from build123d import *

# Parameters (mm, degrees)
SKETCH1_W            = 105
SKETCH1_H            = 85
BOSS_EXTRUDE1_DEPTH  = 3
SKETCH2_W            = 2.8
SKETCH2_H            = 2.8
BOSS_EXTRUDE2_DEPTH  = 15
SKETCH2_7_W          = 7
SKETCH2_7_H          = 7
SKETCH2_7_W_2        = 2.8
SKETCH2_7_H_2        = 2.8
BOSS_EXTRUDE3_DEPTH  = 10
SKETCH4_W            = 2.8
SKETCH4_H            = 2.8
BOSS_EXTRUDE7_DEPTH  = 15
SKETCH8_W            = 7
SKETCH8_H            = 7
SKETCH8_W_2          = 2.8
SKETCH8_H_2          = 2.8
BOSS_EXTRUDE8_DEPTH  = 10
SKETCH9_W            = 2.8
SKETCH9_H            = 2.8
BOSS_EXTRUDE9_DEPTH  = 15
SKETCH10_W           = 7
SKETCH10_H           = 7
SKETCH10_W_2         = 2.8
SKETCH10_H_2         = 2.8
BOSS_EXTRUDE10_DEPTH = 10


with BuildPart() as part:
    # Sketch1 → Boss-Extrude1 (new body)
    with BuildSketch(Plane(origin=(0, 0, 0), x_dir=(1, 0, 0), z_dir=(0, 1, 0))):
        with Locations((-10.290249703, -17.251010702)):
            Rectangle(SKETCH1_W, SKETCH1_H)
    extrude(amount=BOSS_EXTRUDE1_DEPTH)

    # Sketch2 → Boss-Extrude2 (add)
    with BuildSketch(Plane(origin=(0, 3, 0), x_dir=(1, 0, 0), z_dir=(0, 1, 0))):
        with Locations((-24.290249703, -56.430856566)):
            Rectangle(SKETCH2_W, SKETCH2_H)
    extrude(amount=BOSS_EXTRUDE2_DEPTH)

    # Sketch2<7> → Boss-Extrude3 (add)
    with BuildSketch(Plane(origin=(0, 3, 0), x_dir=(1, 0, 0), z_dir=(0, 1, 0))):
        with Locations((-24.290249703, -56.251010702)):
            Rectangle(SKETCH2_7_W, SKETCH2_7_H)
        with Locations((-24.290249703, -56.430856566)):
            Rectangle(SKETCH2_7_W_2, SKETCH2_7_H_2, mode=Mode.SUBTRACT)
    extrude(amount=BOSS_EXTRUDE3_DEPTH)

    # Sketch4 → Boss-Extrude7 (add)
    with BuildSketch(Plane(origin=(0, 3, 0), x_dir=(1, 0, 0), z_dir=(0, 1, 0))):
        with Locations((-24.290249703, 21.748989298)):
            Rectangle(SKETCH4_W, SKETCH4_H)
    extrude(amount=BOSS_EXTRUDE7_DEPTH)

    # Sketch8 → Boss-Extrude8 (add)
    with BuildSketch(Plane(origin=(0, 3, 0), x_dir=(1, 0, 0), z_dir=(0, 1, 0))):
        with Locations((-24.290249703, 21.748989298)):
            Rectangle(SKETCH8_W, SKETCH8_H)
        with Locations((-24.290249703, 21.748989298)):
            Rectangle(SKETCH8_W_2, SKETCH8_H_2, mode=Mode.SUBTRACT)
    extrude(amount=BOSS_EXTRUDE8_DEPTH)

    # Sketch9 → Boss-Extrude9 (add)
    with BuildSketch(Plane(origin=(0, 3, 0), x_dir=(1, 0, 0), z_dir=(0, 1, 0))):
        with Locations((38.709750297, -17.251010702)):
            Rectangle(SKETCH9_W, SKETCH9_H)
    extrude(amount=BOSS_EXTRUDE9_DEPTH)

    # Sketch10 → Boss-Extrude10 (add)
    with BuildSketch(Plane(origin=(0, 3, 0), x_dir=(1, 0, 0), z_dir=(0, 1, 0))):
        with Locations((38.709750297, -17.251010702)):
            Rectangle(SKETCH10_W, SKETCH10_H)
        with Locations((38.709750297, -17.251010702)):
            Rectangle(SKETCH10_W_2, SKETCH10_H_2, mode=Mode.SUBTRACT)
    extrude(amount=BOSS_EXTRUDE10_DEPTH)


solid = part.part
Here's how the part is built. I have some questions about the finished solid (model axes, mm). A direction names the side the tool comes from. Round coordinates to 2 decimals unless told otherwise and drop trailing zeros. Order: outer loops, then holes, each group sorted by start corner. A loop starts at its lowest first (then second) coordinate and runs counter-clockwise, first axis right, second up. Notation, with made-up numbers: (-31, -21.75) -> (-18, -21.75) arc R14 ccw to (-18, -12.75) -> close; hole circle Ø9 at (-17, 81). An arc over 180 degrees is marked (long way). Use CSV: the item, a comma, the result in double quotes.
1. I want a section at C-C on x = -17.5. List the corners of the cut face in (y, z) for me, and give its area (3 significant figures).
Recorded:
outline,"(0, -25.25) -> (3, -25.25) -> (3, 59.75) -> (0, 59.75) -> close"
area,"255 mm2"
2. Thinking about a two-plate mould opening in Z: for faces 6 (the face through (-26, 13, -22)), 7 (the face through (-24, 8, -18.249)), 8 (the face through (-24, 15, -23.149)), 9 (the face through (-11, 0, 17)), which applies, pulls with the +Z half, pulls with the -Z half, needs draft (parallel to the pull), parting line crosses it, or undercut?
Recorded:
face 6,"undercut"
face 7,"undercut"
face 8,"pulls with the -Z half"
face 9,"needs draft"
3. I want a section at B-B on z = 4.5. List the corners of the cut face in (x, y) for me, and give its area (3 significant figures).
Recorded:
outline,"(-62.79, 0) -> (42.21, 0) -> (42.21, 3) -> (-62.79, 3) -> close"
area,"315 mm2"
4. I want a section at A-A on y = 6. List the corners of the cut face in (x, z) for me.
Recorded:
outline,"(-27.79, -25.25) -> (-20.79, -25.25) -> (-20.79, -18.25) -> (-27.79, -18.25) -> close; (-27.79, 52.75) -> (-20.79, 52.75) -> (-20.79, 59.75) -> (-27.79, 59.75) -> close; (35.21, 13.75) -> (42.21, 13.75) -> (42.21, 20.75) -> (35.21, 20.75) -> close"
5. I need wall thicknesses on line 1 along Y through (x, z) = (-1, 14); line 2 along X through (y, z) = (6, 16.5). Which ranges of each line are inside material? Lowest first, please.
Recorded:
line 1,"y = 0 to 3"
line 2,"x = 35.21 to 42.21"
6. Which directions (+Z, -Z, +X, -X, +Y, -Y) give clear straight access to the entire face, cutting with the end or side of a thin tool? Please do faces 1 (the face through (-22.89, 15, 56)), 2 (the face through (42.21, 4, 17)), 3 (the face through (-62.79, 1, 18)), 4 (the face through (39, 15, 15.851)), 5 (the face through (37.31, 15, 17)).
Recorded:
face 1,"+Z, -Z, +X, +Y"
face 2,"+Z, -Z, +X, +Y, -Y"
face 3,"+Z, -Z, -X, +Y, -Y"
face 4,"-Z, +X, -X, +Y"
face 5,"+Z, -Z, -X, +Y"
7. I'm going to push flat-ended pins straight in: P1, Ø3.5, axis at y = 9, z = 57, coming from the +X side; P2, Ø0.8, axis at y = 15.5, z = 57, coming from the +X side; P3, Ø0.8, axis at x = -24.5, y = 15.5, coming from the -Z side. Where does each tip first touch, or does it pass through?
Recorded:
P1,"stops at x = -20.79"
P2,"stops at x = -22.89"
P3,"stops at z = -23.15"
